from build123d import *

# Parameters (mm, degrees)
EXTRUDE_1_DEPTH     = 2
EXTRUDE_2_DEPTH     = 7
EXTRUDE_3_DEPTH     = 5.5
FILLET_1_R          = 2
FILLET_2_R          = 2.5
CUT_EXTRUDE_1_DEPTH = 2.2
SKETCH_7_R          = 0.5
SKETCH_7_R_2        = 0.502126781
CUT_EXTRUDE_2_DEPTH = 0.5


with BuildPart() as part:
    # Эскиз1 → Бобышка-Вытянуть1 (new body)
    with BuildSketch(Plane(origin=(0, 0, 0), x_dir=(1, 0, 0), z_dir=(0, 1, 0))):
        Polygon((-36.5, 28.5), (-36.5, -28.5), (33.96, -28.5), (33.96, -24.788427125), (36.5, -22.248427125), (36.5, 13.174427125), (33.96, 15.714427125), (33.96, 28.5), align=None)
        with BuildLine():
            Line((18.891876357, -26), (-18.891876357, -26))
            ThreePointArc((-18.891876357, -26), (-22.680657515, -23.282629072), (-21.321676788, -18.822568668))
            Line((-21.321676788, -18.822568668), (-2.42980043, -4.375839689))
            ThreePointArc((-2.42980043, -4.375839689), (0, -3.553271021), (2.42980043, -4.375839689))
            Line((2.42980043, -4.375839689), (21.321676788, -18.822568668))
            ThreePointArc((21.321676788, -18.822568668), (22.680657515, -23.282629072), (18.891876357, -26))
        make_face(mode=Mode.SUBTRACT)
        with BuildLine():
            Line((34, 12.138893219), (34, -15.38790545))
            ThreePointArc((34, -15.38790545), (31.772117135, -18.973934014), (27.57019957, -18.565336782))
            Line((27.57019957, -18.565336782), (7.447553982, -3.177431332))
            ThreePointArc((7.447553982, -3.177431332), (5.877354412, 0), (7.447553982, 3.177431332))
            Line((7.447553982, 3.177431332), (27.57019957, 18.565336782))
            ThreePointArc((27.57019957, 18.565336782), (29.443384545, 19.348988538), (31.46, 19.111935525))
            Line((31.46, 19.111935525), (31.46, 14.678893219))
            Line((31.46, 14.678893219), (34, 12.138893219))
        make_face(mode=Mode.SUBTRACT)
        with BuildLine():
            Line((-18.891876357, 26), (18.891876357, 26))
            ThreePointArc((18.891876357, 26), (22.680657515, 23.282629072), (21.321676788, 18.822568668))
            Line((21.321676788, 18.822568668), (2.42980043, 4.375839689))
            ThreePointArc((2.42980043, 4.375839689), (0, 3.553271021), (-2.42980043, 4.375839689))
            Line((-2.42980043, 4.375839689), (-21.321676788, 18.822568668))
            ThreePointArc((-21.321676788, 18.822568668), (-22.680657515, 23.282629072), (-18.891876357, 26))
        make_face(mode=Mode.SUBTRACT)
        with BuildLine():
            Line((-34, -15.38790545), (-34, 15.38790545))
            ThreePointArc((-34, 15.38790545), (-31.772117135, 18.973934014), (-27.57019957, 18.565336782))
            Line((-27.57019957, 18.565336782), (-7.447553982, 3.177431332))
            ThreePointArc((-7.447553982, 3.177431332), (-5.877354412, 0), (-7.447553982, -3.177431332))
            Line((-7.447553982, -3.177431332), (-27.57019957, -18.565336782))
            ThreePointArc((-27.57019957, -18.565336782), (-31.772117135, -18.973934014), (-34, -15.38790545))
        make_face(mode=Mode.SUBTRACT)
    extrude(amount=EXTRUDE_1_DEPTH)

    # Эскиз5 → Бобышка-Вытянуть2 (add)
    with BuildSketch(Plane(origin=(0, 0, 0), x_dir=(1, 0, 0), z_dir=(0, 1, 0))):
        Polygon((33.96, -26.5), (33.96, -28.5), (-36.5, -28.5), (-36.5, 28.5), (31.96, 28.5), (33.96, 28.5), (33.96, 15.714427125), (36.5, 13.174427125), (36.5, -22.248427125), (33.96, -24.788427125), align=None)
        Polygon((31.96, -23.96), (34.5, -21.42), (34.5, 12.346), (31.96, 14.886), (31.96, 26.5), (-34.5, 26.5), (-34.5, -26.5), (31.96, -26.5), align=None, mode=Mode.SUBTRACT)
    extrude(amount=EXTRUDE_2_DEPTH)

    # Эскиз6 → Бобышка-Вытянуть3 (add)
    with BuildSketch(Plane(origin=(0, 0, 0), x_dir=(1, 0, 0), z_dir=(0, 1, 0))):
        Polygon((31.96, -23.96), (31.96, -26.5), (-34.5, -26.5), (-34.5, 26.5), (31.96, 26.5), (31.96, 14.886), (34.5, 12.346), (34.5, -21.42), align=None)
        Polygon((31.46, 26), (-34, 26), (-34, -26), (31.46, -26), (31.46, -23.96), (31.46, -23.752893219), (31.606446609, -23.606446609), (34, -21.212893219), (34, 12.138893219), (31.606446609, 14.532446609), (31.46, 14.678893219), (31.46, 14.886), align=None, mode=Mode.SUBTRACT)
    extrude(amount=EXTRUDE_3_DEPTH)

    # Скругление1
    fillet_1_edges = [part.edges().sort_by_distance(p)[0] for p in [
        (31.96, 6.25, 23.96),
        (31.96, 6.25, -14.886),
        (33.96, 3.5, 28.5),
        (-36.5, 3.5, 28.5),
        (-36.5, 3.5, -28.5),
        (33.96, 3.5, -28.5),
        (36.5, 3.5, -13.174427125),
        (36.5, 3.5, 22.248427125),
    ]]
    fillet(fillet_1_edges, radius=FILLET_1_R)

    # Скругление2
    fillet_2_edges = [part.edges().sort_by_distance(p)[0] for p in [
        (31.46, 3.75, 23.752893219),
        (31.46, 2.75, -14.678893219),
    ]]
    fillet(fillet_2_edges, radius=FILLET_2_R)

    # Эскиз4 → Вырез-Вытянуть1 (cut)
    with BuildSketch(Plane(origin=(36.5, 0, 0), x_dir=(0, 0, -1), z_dir=(1, 0, 0))):
        with BuildLine():
            Line((-23.080914643, 0), (-19.962989622, 1.084044193))
            ThreePointArc((-19.962989622, 1.084044193), (-16.346249259, 1.410725958), (-13, 0))
            Line((-13, 0), (-23.080914643, 0))
        make_face()
    cut_extrude_1 = extrude(amount=-CUT_EXTRUDE_1_DEPTH, mode=Mode.SUBTRACT)

    # Зеркальное отражение1: Вырез-Вытянуть1 across plane
    add(cut_extrude_1.mirror(Plane(origin=(0, 0, 0), x_dir=(0, 0, 1), z_dir=(1, 0, 0))), mode=Mode.SUBTRACT)

    # Эскиз7 → Вырез-Вытянуть2 (cut)
    with BuildSketch(Plane.XZ):
        with Locations(Location((14.24363767, 9.937218253, 0), (0, 0, 270))):
            Circle(SKETCH_7_R)
        with Locations(Location((23.6, -26.1, 0), (0, 0, 270))):
            Circle(SKETCH_7_R)
        with Locations(Location((-14.24363767, 9.937218253, 0), (0, 0, 270))):
            Circle(SKETCH_7_R)
        with Locations(Location((-23.6, -26.1, 0), (0, 0, 270))):
            Circle(SKETCH_7_R_2)
    extrude(amount=-CUT_EXTRUDE_2_DEPTH, mode=Mode.SUBTRACT)


solid = part.part
The listing builds one solid part. Answer for the finished solid, in the listing's coordinates (mm). A direction names the side the tool comes from. Give positions to 0.01 mm unless a question says otherwise; leave off trailing zeros. Order: outer loops, then holes, each group sorted by start corner. A loop starts at its lowest first (then second) coordinate and runs counter-clockwise, first axis right, second up. Notation, with made-up numbers: (39.25, -30.5) -> (58.25, -30.5) arc R20 cw to (58.25, -17.5) -> close; hole circle Ø10 at (-7.75, 5.25). An arc over 180 degrees is marked (long way). Put each result on its own line as item: value.
Item 1: A cutting plane is placed at A-A on z = 5.5. Give the vertices of the cut face in (x, y), plus the area to 3 significant figures.
Established:
outline: (-36.5, 0) -> (-34, 0) -> (-34, 5.5) -> (-34.5, 5.5) -> (-34.5, 7) -> (-36.5, 7) -> close; (-10.48, 0) -> (-3.9, 0) -> (-3.9, 2) -> (-10.48, 2) -> close; (3.9, 0) -> (10.48, 0) -> (10.48, 2) -> (3.9, 2) -> close; (34, 0) -> (36.5, 0) -> (36.5, 7) -> (34.5, 7) -> (34.5, 5.5) -> (34, 5.5) -> close
area: 59.8 mm^2
Item 2: For faces 4 (the face through (31.46, 3, -21)), 5 (the face through (31.645, 1.014, -14.77)), 6 (the face through (34.923, 3.451, 23.825)), determine the directions among +Z, -Z, +X, -X, +Y, -Y from which every point of the face is accessible in a straight line to the end or side of a thin tool.
Established:
face 4: +Y
face 5: +Y, -Y
face 6: +Z, +X, +Y, -Y
Item 3: Given P1, Ø0.5, axis at x = 23.5, z = -26, coming from the -Y side; P2, Ø1.2, axis at y = 0.5, z = 17.5, coming from the +X side, each flat-ended and moving along its own axis, determine where each tip first touches the part or whether it passes through.
Established:
P1: stops at y = 0.5
P2: stops at x = 34.3
Item 4: For a pull along Z with two mould halves and no side action, classify faces 1 (the face through (34.3, 1, 18)), 2 (the face through (33.39, 3.55, 27.9)), 3 (the face through (-35.42, 1.42, 16.4)) as released by +Z, released by -Z, zero draft, split by the parting line, or undercut.
Established:
face 1: undercut
face 2: released by +Z
face 3: undercut
Item 5: Straight lines are drawn through the part: line 1 (Z direction, x = -32, y = 3); line 2 (X direction, y = 0.75, z = -10.5); line 3 (X direction, y = 6.5, z = 19.5). For each, find the intervals that lie inside material, in ascending order.
Established:
line 1: z = -28.5 to -26, 26 to 28.5
line 2: x = -36.5 to -34, -17.02 to -10.44, 10.44 to 17.02, 34 to 36.5
line 3: x = -36.5 to -34.5, 34.5 to 36.5
